from build123d import *

# Parameters (mm, degrees)
F2_R     = 2.5
F3_DEPTH = 5
F4_R     = 2
F5_DEPTH = 25


with BuildPart() as f1:
    # F0 (on Right) → F1 (revolve)
    with BuildSketch(Plane.YZ):
        Polygon((-9.882553, 0), (0, 0), (0, 15), (-16, 15), align=None)
    revolve(axis=Axis((0, 0, 7.5), (0, 0, -1)))

    # F2 (on face) → F3 (cut)
    with BuildSketch(Plane(origin=(0, 0, 0), x_dir=(1, 0, 0), z_dir=(0, 0, -1))):
        Circle(F2_R)
    extrude(amount=-F3_DEPTH, mode=Mode.SUBTRACT)

    # F4 (on face) → F5 (cut)
    with BuildSketch(Plane.XY.offset(15)):
        Circle(F4_R)
    extrude(amount=-F5_DEPTH, mode=Mode.SUBTRACT)


solid = f1.part
Here's how the part is built. I have some questions about the finished solid (model axes, mm). A direction names the side the tool comes from. Coordinates: 2 decimals unless noted, no trailing zeros. Write each loop counter-clockwise with the first axis right and the second up, starting at its lowest first coordinate (ties: lowest second). Pieces come first, ordered by that corner, then holes.
Item 1: I want a section at C-C on z = 7. Write out the boundary of the cut face in (x, y), and give its area (3 significant figures).
Item 2: On a 3-axis mill with a long thin cutter (end or side, diameter ignored), from which of +Z, -Z, +X, -X, +Y, -Y can I reach the whole of each face in a straight line? I mean faces 5 (the flat face through (3, 0, 15)), 6 (the flat face through (-1, -2, 5)). Say none if no direction works.
Item 3: If we mould it in two halves opening along X, with no side actions, what happens to faces 1 (the cylindrical face through (0, -2, 10)), 2 (the cylindrical face through (-0.54, 2.44, 2.46)), 3 (the flat face through (2, -2, 0)), 4 (the conical face through (10.601, 2.354, 2.395))? For each: +X half, -X half, draft (parallel to the pull), parting line (faces both ways), or undercut.
Item 4: If I drill on line 1 (X direction, y = 0, z = 3.85); line 2 (Y direction, x = 1.5, z = 10.75); line 3 (X direction, y = 1.5, z = 2), over which ranges is the centre line in solid material (lowest first)?
Item 5: I want a section at A-A on x = 0. Write out the boundary of the cut face in (y, z), and give its area (3 significant figures).
Item 6: I want a section at D-D on z = 9. Write out the boundary of the cut face in (x, y).
Item 7: Will this pin go through, and if not, where does the flat tip stop? pin 1 (2 mm diameter, centred on x = 10, y = 12, fed in from -Z).
Findings below:
1. outline: circle Ø25.47 at (0, 0); hole circle Ø4 at (0, 0)
1. area: 497 mm2
2. face 5: +Z, +X, -X, +Y, -Y
2. face 6: -Z
3. face 1: undercut
3. face 2: undercut
3. face 3: draft
3. face 4: parting line
4. line 1: x = -11.45 to -2.5, 2.5 to 11.45
4. line 2: y = -14.19 to -1.32, 1.32 to 14.19
4. line 3: x = -10.59 to -2, 2 to 10.59
5. outline: (-16, 15) - (-9.88, 0) - (-2.5, 0) - (-2.5, 5) - (-2, 5) - (-2, 15) - close; (2, 5) - (2.5, 5) - (2.5, 0) - (9.88, 0) - (16, 15) - (2, 15) - close
5. area: 323 mm2
6. outline: circle Ø27.11 at (0, 0); hole circle Ø4 at (0, 0)
7. pin 1: stops at z = 11.62
